The model under review builds one solid part; all positions refer to its coordinate system, in mm. Round coordinates to 2 decimals unless told otherwise and drop trailing zeros. Answer as a JSON object with one key per item and string values. Group by question number.
1) Insertion check: pin 1 Ø1.5 at (x, y) = (30, 126) entering from -Z. The pin has a flat end and moves straight along its axis. Give the tip position at first contact, or say it passes through.
2) To check wall thickness, follow probe 1 along Y at (x, z) = (51, 1750); probe 2 along Z at (x, y) = (59, 85); probe 3 along Z at (x, y) = (52.5, 99). State the ranges of each line that lie inside material, in increasing order. Write a range as [from, to].
3) Mouldability with a two-part tool opening along Z and no side actions: class faces 1 (the flat face through (-1, 88, 0)), 2 (the flat face through (-65, 88, 986)), 3 (the cylindrical face through (39.65, 89.26, 1769.83)), 4 (the conical face through (5.07, 86.201, 1753.444)) as pulls with the +Z half, pulls with the -Z half, needs draft (parallel to the pull), parting line crosses it, or undercut.
from build123d import *

# Parameters (mm, degrees)
F1_DEPTH = 2000
F3_D     = 40
F3_DEPTH = 50
F3_TIP   = 12.0172123806


with BuildPart() as f1:
    # F0 (on Top) → F1 (new body)
    with BuildSketch(Plane.XY):
        Polygon((-34.2555230263, 181.6535690603), (-65, 181.6535690603), (-65, -8.3464309397), (65, -8.3464309397), (65, 181.6535690603), (34.2555230263, 181.6535690603), align=None)
    extrude(amount=F1_DEPTH)

    # F3
    with Locations(Plane.YZ.offset(65)):
        with Locations((86.6535690603, 1750)):
            Hole(F3_D / 2, depth=F3_DEPTH)
            with Locations((0, 0, -(F3_DEPTH + F3_TIP / 2))):  # 118° drill point
                Cone(0, F3_D / 2, F3_TIP, mode=Mode.SUBTRACT)


solid = f1.part
Here are the results:
{
 "1": {"pin 1": "stops at z = 0"},
 "2": {"probe 1": "y = [-8.35, 66.65], [106.65, 181.65]", "probe 2": "z = [0, 1730.07], [1769.93, 2000]", "probe 3": "z = [0, 1734.27], [1765.73, 2000]"},
 "3": {"face 1": "pulls with the -Z half", "face 2": "needs draft", "face 3": "undercut", "face 4": "undercut"}
}
